The listing builds one solid part. Answer for the finished solid, in the listing's coordinates (mm). A direction names the side the tool comes from. Round coordinates to 2 decimals unless told otherwise and drop trailing zeros. Write each loop counter-clockwise with the first axis right and the second up, starting at its lowest first coordinate (ties: lowest second). Pieces come first, ordered by that corner, then holes. Notation, with made-up numbers: (14, 31) - (49, 31) arc R18 cw to (49, 46) - close; hole circle Ø3 at (36, 0). An arc over 180 degrees is marked (long way). Use a Markdown table: item, result. Add a question column.
1) Determine the mould class of faces 3 (the cylindrical face through (32, 2, -1)), 4 (the cylindrical face through (2.354, 34.616, 0.774)), 5 (the flat face through (26, 0, 3)), 6 (the cylindrical face through (49.364, 3.413, 0.156)) for opening direction Y: +Y half, -Y half, draft (parallel to the pull), parting line (faces both ways), or undercut.
2) A cutting plane is placed at D-D (z = -4.75). Give the vertices of the cut face in (x, y) (3 decimals), then the cut area to 3 significant figures.
3) Each of these flat-tipped pins is pushed along its axis until it touches: P1, Ø1.5, axis at y = 21.5, z = 0, coming from the +X side (3 decimals); P2, Ø11, axis at y = 29.5, z = 4.5, coming from the +X side; P3, Ø11, axis at x = 18, z = 5.5, coming from the +Y side. Where does it stop, or does it pass through?
4) A tool of negligible diameter and unlimited length cuts with its end or side. For faces 1 (the flat face through (14, 3, 11.112)), 2 (the flat face through (22, 4.775, 0)), from which of +Z, -Z, +X, -X, +Y, -Y can it reach the whole face along a straight path? Write none if from no direction.
5) A cutting plane is placed at B-B (z = 0). Give the vertices of the cut face in (x, y) (3 decimals).
6) A cutting plane is placed at A-A (y = 19.05). Give the vertices of the cut face in (x, z).
7) A cutting plane is placed at C-C (x = 4). Give the vertices of the cut face in (y, z).
8) Find the intervals of material crossed by probe 1 along Y at (x, z) = (1.15, 0); probe 2 along Z at (x, y) = (1, 38.1); probe 3 along Y at (x, z) = (15, -6.25), in increasing order. Write a range as from..to.
```python
from build123d import *

# Parameters (mm, degrees)
BOSS_EXTRUDE1_DEPTH = 11.1125
SKETCH2_R           = 3.5687
CUT_EXTRUDE1_DEPTH  = 51.8
SKETCH3_R           = 3.5687
CUT_EXTRUDE2_DEPTH  = 51.8


with BuildPart() as part:
    # Sketch1 → Boss-Extrude1 (new body, symmetric)
    with BuildSketch(Plane.XY):
        with BuildLine():
            Line((0, 0), (0, 50.8))
            ThreePointArc((0, 50.8), (3.376576302, 49.401376302), (4.7752, 46.0248))
            Line((4.7752, 46.0248), (4.7752, 7.9502))
            ThreePointArc((4.7752, 7.9502), (5.70513597, 5.70513597), (7.9502, 4.7752))
            Line((7.9502, 4.7752), (46.0248, 4.7752))
            ThreePointArc((46.0248, 4.7752), (49.401376302, 3.376576302), (50.8, 0))
            Line((50.8, 0), (0, 0))
        make_face()
    extrude(amount=BOSS_EXTRUDE1_DEPTH, both=True)

    # Sketch2 → Cut-Extrude1 (cut, through all)
    with BuildSketch(Plane(origin=(0, 0, 0), x_dir=(1, 0, 0), z_dir=(0, 1, 0))):
        with Locations((28.575, 0)):
            Circle(SKETCH2_R)
    extrude(amount=CUT_EXTRUDE1_DEPTH, mode=Mode.SUBTRACT)

    # Sketch3 → Cut-Extrude2 (cut, through all)
    with BuildSketch(Plane(origin=(0, 0, 0), x_dir=(0, 0, -1), z_dir=(1, 0, 0))):
        with Locations((0, 19.05)):
            Circle(SKETCH3_R)
        with Locations((0, 38.1)):
            Circle(SKETCH3_R)
    extrude(amount=CUT_EXTRUDE2_DEPTH, mode=Mode.SUBTRACT)


solid = part.part
```
Entries:
| question | item | result |
|---|---|---|
| 1 | face 3 | draft |
| 1 | face 4 | undercut |
| 1 | face 5 | -Y half |
| 1 | face 6 | +Y half |
| 2 | outline | (0, 0) - (50.8, 0) arc R4.775 ccw to (46.025, 4.775) - (7.95, 4.775) arc R3.175 cw to (4.775, 7.95) - (4.775, 46.025) arc R4.775 ccw to (0, 50.8) - close |
| 2 | area | 455 mm² |
| 3 | P1 | passes through |
| 3 | P2 | stops at x = 4.78 |
| 3 | P3 | stops at y = 4.78 |
| 4 | face 1 | +Z, +X, -X, +Y, -Y |
| 4 | face 2 | +Z, -Z, +X, +Y |
| 5 | outline | (0, 0) - (25.006, 0) - (25.006, 4.775) - (7.95, 4.775) arc R3.175 cw to (4.775, 7.95) - (4.775, 15.481) - (0, 15.481) - close; (0, 22.619) - (4.775, 22.619) - (4.775, 34.531) - (0, 34.531) - close; (0, 41.669) - (4.775, 41.669) - (4.775, 46.025) arc R4.775 ccw to (0, 50.8) - close; (32.144, 0) - (50.8, 0) arc R4.775 ccw to (46.025, 4.775) - (32.144, 4.775) - close |
| 6 | outline | (0, -11.11) - (4.78, -11.11) - (4.78, -3.57) - (0, -3.57) - close; (0, 3.57) - (4.78, 3.57) - (4.78, 11.11) - (0, 11.11) - close |
| 7 | outline | (0, -11.11) - (48.63, -11.11) - (48.63, 11.11) - (0, 11.11) - close; hole circle Ø7.14 at (19.05, 0); hole circle Ø7.14 at (38.1, 0) |
| 8 | probe 1 | y = 0..15.48, 22.62..34.53, 41.67..50.66 |
| 8 | probe 2 | z = -11.11..-3.57, 3.57..11.11 |
| 8 | probe 3 | y = 0..4.78 |
